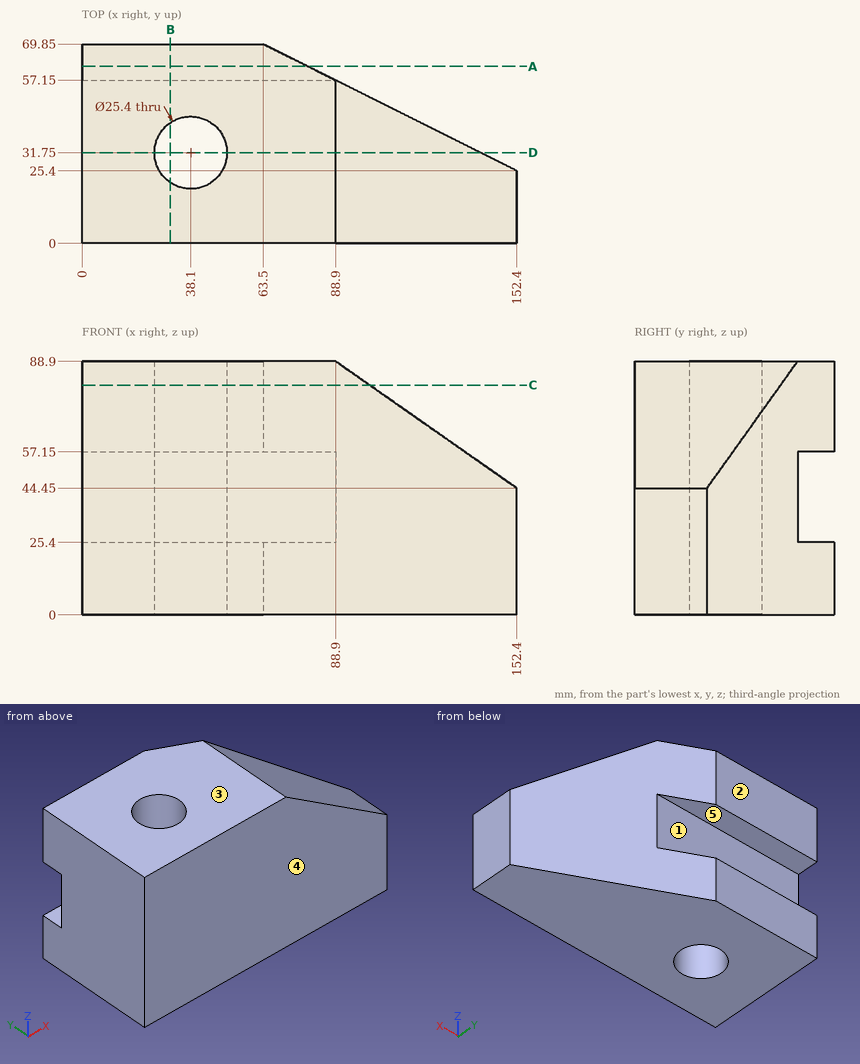
The figure shows three views and two pictorial views of one solid part (mm, origin at its lowest corner). Answer the questions. A direction names the side the tool comes from. Round coordinates to 2 decimals unless told otherwise and drop trailing zeros. Order: outer loops, then holes, each group sorted by start corner. A loop starts at its lowest first (then second) coordinate and runs counter-clockwise, first axis right, second up. Notation, with made-up numbers: (-21, 89) -> (34, 89) arc R29 ccw to (34, 111) -> close; hole circle Ø2 at (59, 23.5). An arc over 180 degrees is marked (long way). Put each result on its own line as item: value.
Q1. Section C-C, the plane z = 80.5 is taken. Write down the section's boundary in (x, y), and give its area (3 significant figures).
Results list:
outline: (0, 0) -> (100.9, 0) -> (100.9, 51.15) -> (63.5, 69.85) -> (0, 69.85) -> close; hole circle Ø25.4 at (38.1, 31.75)
area: 6,190 mm^2
Q2. Section D-D, the plane y = 31.75 is taken. Write down the section's boundary in (x, z), and give its area (3 significant figures).
Results list:
outline: (0, 0) -> (25.4, 0) -> (25.4, 88.9) -> (0, 88.9) -> close; (50.8, 0) -> (139.7, 0) -> (139.7, 53.34) -> (88.9, 88.9) -> (50.8, 88.9) -> close
area: 9,260 mm^2
Q3. Consider line 1 along Z through (x, y) = (26.5, 63.5); line 2 along Y through (x, z) = (38.1, 23); line 3 along Y through (x, z) = (38.1, 38). Determine where each line is inside the solid, lowest interval first.
Results list:
line 1: 0 to 25.4, 57.15 to 88.9
line 2: 0 to 19.05, 44.45 to 69.85
line 3: 0 to 19.05, 44.45 to 57.15
Q4. Section A-A, the plane y = 62 is taken. Write down the section's boundary in (x, z).
Results list:
outline: (0, 0) -> (79.2, 0) -> (79.2, 25.4) -> (0, 25.4) -> close; (0, 57.15) -> (79.2, 57.15) -> (79.2, 88.9) -> (0, 88.9) -> close
Q5. Determine the mould class of the marked faces 1, 2 and 3 for opening direction Z: pulls with the +Z half, pulls with the -Z half, needs draft (parallel to the pull), parting line crosses it, or undercut.
Results list:
face 1: undercut
face 2: needs draft
face 3: pulls with the +Z half
Q6. Which of the six approach directions +Z, -Z, +X, -X, +Y, -Y give full straight-line access (tool end or side, diameter ignored) to the marked faces 4 and 5?
Results list:
face 4: +Z, -Z, +X, -X, -Y
face 5: +X, -X, +Y
Q7. Each of these flat-tipped pins is pushed along its axis until it touches: P1, Ø5, axis at x = 73, z = 10, coming from the +Y side; P2, Ø23, axis at x = 38.1, y = 31.75, coming from the +Z side; P3, Ø1.5, axis at y = 21, z = 64, coming from the +X side; P4, Ø10, axis at x = 88, z = 52, coming from the +Y side. Where does it stop, or does it pass through?
Results list:
P1: y = 66.35
P2: through
P3: x = 125.54
P4: y = 57.15
Q8. Section B-B, the plane x = 31 is taken. Write down the section's boundary in (y, z).
Results list:
outline: (0, 0) -> (21.22, 0) -> (21.22, 88.9) -> (0, 88.9) -> close; (42.28, 0) -> (69.85, 0) -> (69.85, 25.4) -> (57.15, 25.4) -> (57.15, 57.15) -> (69.85, 57.15) -> (69.85, 88.9) -> (42.28, 88.9) -> close
